Geometry: final body of the model. Coordinates: model frame, mm. Face numbers are marked on the shaded views. A direction names the side the tool comes from. Round coordinates to 2 decimals unless told otherwise and drop trailing zeros. Write each loop counter-clockwise with the first axis right and the second up, starting at its lowest first coordinate (ties: lowest second). Pieces come first, ordered by that corner, then holes. Notation, with made-up numbers: M 6.25,53 L 29.25,53 A14 cw 29.25,67 Z; hole C 9,50.5 d8. An arc over 180 degrees is marked long. Answer as CSV lines item,"result". Start each with the question number.
Q1. Section query A-A on z = -14.5. Output: boundary loops of the cut face in (x, y).
Q2. Section query C-C on z = -12. Output: boundary loops of the cut face in (x, y).
Q3. Ray query, probe 1 along X at (y, z) = (0.4, -17.25); probe 2 along X at (y, z) = (0.7, -20.25); probe 3 along Z at (x, y) = (-38.5, 0.5). Return the intervals inside material, ascending.
Q4. Section query B-B on y = 1.8. Give the number of separate pieces and of enclosed holes in the cut face, and give its area (3 significant figures).
Q5. Reachability of the marked faces 5 and 6 from +Z, -Z, +X, -X, +Y, -Y: full face, straight path, thin tool, end or side. Return the list, or none.
Q6. Mould query, pull axis Z, two halves, no side actions, for the marked faces 1, 2, 3 and 4. Classes: pulls with the +Z half, pulls with the -Z half, needs draft (parallel to the pull), parting line crosses it, or undercut.
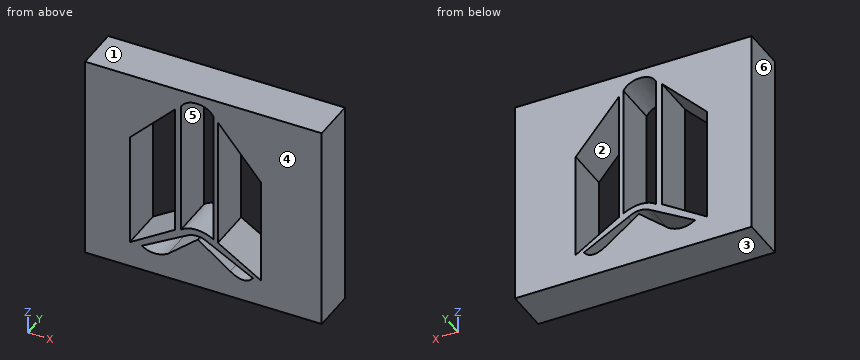
```python
from build123d import *

# Parameters (mm, degrees)
SKETCH2_W           = 16
SKETCH2_H           = 14
BOSS_EXTRUDE1_DEPTH = 3
CUT_EXTRUDE1_DEPTH  = 3


with BuildPart() as part:
    # Sketch2 → Boss-Extrude1 (new body)
    with BuildSketch(Plane(origin=(0, 0, 0), x_dir=(1, 0, 0), z_dir=(0, 1, 0))):
        with Locations((-34.802547771, 15.318471338)):
            Rectangle(SKETCH2_W, SKETCH2_H)
    extrude(amount=BOSS_EXTRUDE1_DEPTH)

    # Sketch4 → Cut-Extrude1 (cut)
    with BuildSketch(Plane(origin=(0, 3, 0), x_dir=(1, 0, 0), z_dir=(0, 1, 0))):
        with BuildLine():
            Line((-36.318911755, 18.516121759), (-36.318911755, 9.495766822))
            add(Edge.make_bspline(
                [(-36.318911755, 9.495766822), (-35.913871603, 8.720893634), (-34.543281821, 8.741015584), (-34.130046647, 9.495766822)],
                knots=[0, 0, 0, 0, 1, 1, 1, 1], degree=3))
            Line((-34.130046647, 9.495766822), (-34.130046647, 18.516121759))
            add(Edge.make_bspline(
                [(-36.318911755, 18.516121759), (-35.70959357, 18.038988867), (-34.764466339, 18.114801672), (-34.130046647, 18.516121759)],
                knots=[0, 0, 0, 0, 1, 1, 1, 1], degree=3))
        make_face()
        Polygon((-33.822053837, 18.666521758), (-33.822053837, 9.831273412), (-30.905859423, 13.283968712), (-30.905859423, 20.48178763), align=None)
        Polygon((-36.726560822, 18.666521758), (-36.726560822, 9.831273412), (-39.779226537, 12.883939127), (-39.779226537, 20.575922696), align=None)
        with BuildLine():
            Line((-37.197236152, 20.575922696), (-35.179234522, 18.871490486))
            Line((-35.179234522, 18.871490486), (-35.103321149, 18.927279173))
            Line((-35.103321149, 18.927279173), (-32.988053911, 20.48178763))
            add(Edge.make_bspline(
                [(-32.988053911, 20.48178763), (-31.996391296, 21.194388002), (-31.454997121, 20.48178763)],
                knots=[0, 0, 0, 1, 1, 1], degree=2))
            Line((-31.454997121, 20.48178763), (-34.453871369, 18.871490486))
            add(Edge.make_bspline(
                [(-36.013823893, 18.871490486), (-35.223935459, 18.378867512), (-34.453871369, 18.871490486)],
                knots=[0, 0, 0, 1, 1, 1], degree=2))
            Line((-36.013823893, 18.871490486), (-38.972354542, 20.575922696))
            add(Edge.make_bspline(
                [(-38.972354542, 20.575922696), (-38.119189313, 21.114619825), (-37.197236152, 20.575922696)],
                knots=[0, 0, 0, 1, 1, 1], degree=2))
        make_face()
    extrude(amount=-CUT_EXTRUDE1_DEPTH, mode=Mode.SUBTRACT)


solid = part.part
```
Entries:
1,outline,"M -42.8,0 L -39.78,0 L -39.78,3 L -42.8,3 Z; M -36.73,0 L -36.32,0 L -36.32,3 L -36.73,3 Z; M -34.13,0 L -33.82,0 L -33.82,3 L -34.13,3 Z; M -30.91,0 L -26.8,0 L -26.8,3 L -30.91,3 Z"
2,outline,"M -42.8,0 L -38.9,0 L -38.9,3 L -42.8,3 Z; M -36.73,0 L -36.32,0 L -36.32,3 L -36.73,3 Z; M -34.13,0 L -33.82,0 L -33.82,3 L -34.13,3 Z; M -31.99,0 L -26.8,0 L -26.8,3 L -31.99,3 Z"
3,probe 1,"x = -42.8 to -39.78, -36.73 to -36.32, -34.13 to -33.82, -30.91 to -26.8"
3,probe 2,"x = -42.8 to -39.78, -39.26 to -38.41, -36.81 to -33.3, -31.89 to -31.28, -30.91 to -26.8"
3,probe 3,"z = -22.32 to -20.79, -20.3 to -19.78, -11.6 to -8.32"
4,separate pieces,"1"
4,enclosed holes,"4"
4,area,"150 mm^2"
5,face 5,"+Y, -Y"
5,face 6,"+Z, -Z, -X, +Y, -Y"
6,face 1,"pulls with the +Z half"
6,face 2,"undercut"
6,face 3,"pulls with the -Z half"
6,face 4,"needs draft"
